Work out the finished part from the listing and answer in its coordinate system (mm). Round coordinates to 2 decimals unless told otherwise and drop trailing zeros. Loops run counter-clockwise (first coordinate to the right, second up) from the corner with the lowest first, then second, coordinate; pieces in that order, holes last. Notation, with made-up numbers: M -12,44.5 L 38,44.5 A9 ccw 38,61.5 Z; hole C 9.5,2.5 d7. An arc over 180 degrees is marked long. One line per item, written item: value.
```python
from build123d import *

# Parameters (mm, degrees)
F0_W     = 3.12686
F0_H     = 3.290719
F1_DEPTH = 38.1


with BuildPart() as f1:
    # F0 (on Top) → F1 (new body)
    with BuildSketch(Plane.XY):
        with BuildLine():
            Line((-90.932, 0), (-94.22225, 0))
            ThreePointArc((-94.22225, 0), (-67.175674, -66.070124), (-1.56343, -94.209278))
            Line((-1.56343, -94.209278), (-1.56343, -90.918559))
            ThreePointArc((-1.56343, -90.918559), (-64.849034, -63.743481), (-90.932, 0))
        make_face()
        with Locations((0, -92.563918)):
            Rectangle(F0_W, F0_H)
        with BuildLine():
            Line((1.56343, -90.918559), (1.56343, -94.209278))
            ThreePointArc((1.56343, -94.209278), (67.175674, -66.070124), (94.22225, 0))
            Line((94.22225, 0), (90.932, 0))
            ThreePointArc((90.932, 0), (64.849034, -63.743481), (1.56343, -90.918559))
        make_face()
    extrude(amount=F1_DEPTH)


solid = f1.part
```
1) Find section B-B (z = 4). Give the vertices of the cut face in (x, y), then the cut area to 3 significant figures.
Check values:
outline: M -94.22,0 A94.22 ccw -1.56,-94.21 L 1.56,-94.21 A94.22 ccw 94.22,0 L 90.93,0 A90.93 cw 1.56,-90.92 L -1.56,-90.92 A90.93 cw -90.93,0 Z
area: 957 mm2
2) Each of these flat-tipped pins is pushed along its axis until it touches: pin 1 (1.5 mm diameter, centred on y = -55.5, z = 13.5, fed in from +X); pin 2 (2.5 mm diameter, centred on x = -0.5, z = 11.5, fed in from +Y); pin 3 (10 mm diameter, centred on y = -57.5, z = 10.5, fed in from -X). Where does it stop, or does it pass through?
Check values:
pin 1: x = 76.68
pin 2: y = -90.92
pin 3: x = -78.24
3) Find section C-C (y = -89). Give the vertices of the cut face in (x, z).
Check values:
outline: M -30.93,0 L -18.64,0 L -18.64,38.1 L -30.93,38.1 Z; M 18.64,0 L 30.93,0 L 30.93,38.1 L 18.64,38.1 Z
4) Find the intervals of material crossed by probe 1 along Y at (x, z) = (1, 26.5); probe 2 along X at (y, z) = (-55.5, 9.5); probe 3 along X at (y, z) = (-6.5, 31.5), in increasing order. Write a range as from..to.
Check values:
probe 1: -94.21..-90.92
probe 2: -76.14..-72.03, 72.03..76.14
probe 3: -94..-90.7, 90.7..94
5) The mould has two halves that part along X. Classify faces 1 (the face through (-7, -92, 0)), 2 (the face through (66.45, -66.8, 18.78)), 3 (the face through (-64.152, -64.445, 18.783)), 4 (the face through (65.54, -63.03, 18.78)): +X half, -X half, draft (parallel to the pull), parting line (faces both ways), or undercut.
Check values:
face 1: draft
face 2: +X half
face 3: undercut
face 4: undercut
6) Find section D-D (x = -76). Give the vertices of the cut face in (y, z), then the cut area to 3 significant figures.
Check values:
outline: M -55.69,0 L -49.93,0 L -49.93,38.1 L -55.69,38.1 Z
area: 220 mm2
7) Find section A-A (y = -67). Give the vertices of the cut face in (x, z), then the cut area to 3 significant figures.
Check values:
outline: M -66.25,0 L -61.48,0 L -61.48,38.1 L -66.25,38.1 Z; M 61.48,0 L 66.25,0 L 66.25,38.1 L 61.48,38.1 Z
area: 363 mm2
